Build history of the part. All positions in model axes, mm. A direction names the side the tool comes from. Round coordinates to 2 decimals unless told otherwise and drop trailing zeros. Write each loop counter-clockwise with the first axis right and the second up, starting at its lowest first coordinate (ties: lowest second). Pieces come first, ordered by that corner, then holes.
Item 1: Band-saw the part on C-C, the plane y = -17. Write the cut outline in (x, z), then the cut area to 3 significant figures.
Item 2: Band-saw the part on D-D, the plane y = -1.5. Write the cut outline in (x, z).
Item 3: 3-axis set-ups, long thin cutter, end or side, ignore diameter. For faces 1 (the flat face through (-19.198, 6, -4)), 2 (the flat face through (5, -15.387, 25)), 3 (the flat face through (-16.698, 7, 25)), 4 (the flat face through (7, 9, 0)): which of +Z, -Z, +X, -X, +Y, -Y reach the whole face in a straight line?
Item 4: Mould opens along Y. For faces 5 (the flat face through (7, -12.887, 25)), 6 (the flat face through (-21.698, 4, 22)), 7 (the flat face through (5, -17.887, 25)) say: +Y half, -Y half, draft (parallel to the pull), parting line (faces both ways), or undercut.
Item 5: Drop flat-ended pins along their axis: pin 1 Ø21 at (y, z) = (7.5, 24.5) entering from +X; pin 2 Ø24 at (x, y) = (0, 11.5) entering from +Z; pin 3 Ø1.2 at (y, z) = (13.5, -4) entering from +X. Give the stop position or say it passes through.
Item 6: Band-saw the part on B-B, the plane x = -8. Write the cut outline in (y, z).
Item 7: Band-saw the part on A-A, the plane z = 38. Write the cut outline in (x, y), then the cut area to 4 significant figures.
Item 8: Wall check: probe 1 along Y at (x, z) = (9, 21.5); probe 2 along Z at (x, y) = (8.5, 0.5); probe 3 along X at (y, z) = (6, 41). Give the ranges that are in metal, low to high.
```python
from build123d import *

# Parameters (mm, degrees)
F0_W     = 42.5
F0_H     = 42.5
F0_W_2   = 2.5
F0_H_2   = 2.5
F1_DEPTH = 2.5
F2_DEPTH = 50
F3_W     = 2.5
F3_H     = 47.5
F3_W_2   = 47.5
F3_H_2   = 2.5
F4_DEPTH = 2.5
F5_W     = 47.5
F5_H     = 47.5
F6_DEPTH = 2.5


with BuildPart() as f1:
    # F0 (on Top) → F1 (new body)
    with BuildSketch(Plane.XY):
        with Locations((7.0520306379, 8.3629446477)):
            Rectangle(F0_W, F0_H)
        with Locations((-15.4479693621, 8.3629446477)):
            Rectangle(F0_W_2, F0_H)
        with Locations((-17.9479693621, 8.3629446477)):
            Rectangle(F0_W_2, F0_H)
        with Locations((-20.4479693621, 8.3629446477)):
            Rectangle(F0_W_2, F0_H)
        with Locations((7.0520306379, -14.1370553523)):
            Rectangle(F0_W, F0_H_2)
        with Locations((7.0520306379, -16.6370553523)):
            Rectangle(F0_W, F0_H_2)
        with Locations((7.0520306379, -19.1370553523)):
            Rectangle(F0_W, F0_H_2)
        with Locations((-15.4479693621, -19.1370553523)):
            Rectangle(F0_W_2, F0_H_2)
        with Locations((-17.9479693621, -19.1370553523)):
            Rectangle(F0_W_2, F0_H_2)
        with Locations((-20.4479693621, -19.1370553523)):
            Rectangle(F0_W_2, F0_H_2)
        with Locations((-20.4479693621, -16.6370553523)):
            Rectangle(F0_W_2, F0_H_2)
        with Locations((-17.9479693621, -16.6370553523)):
            Rectangle(F0_W_2, F0_H_2)
        with Locations((-15.4479693621, -16.6370553523)):
            Rectangle(F0_W_2, F0_H_2)
        with Locations((-15.4479693621, -14.1370553523)):
            Rectangle(F0_W_2, F0_H_2)
        with Locations((-17.9479693621, -14.1370553523)):
            Rectangle(F0_W_2, F0_H_2)
        with Locations((-20.4479693621, -14.1370553523)):
            Rectangle(F0_W_2, F0_H_2)
    extrude(amount=-F1_DEPTH)

    # F0 (on Top) → F2 (join)
    with BuildSketch(Plane.XY):
        with Locations((-20.4479693621, 8.3629446477)):
            Rectangle(F0_W_2, F0_H)
        with Locations((-20.4479693621, -14.1370553523)):
            Rectangle(F0_W_2, F0_H_2)
        with Locations((-15.4479693621, 8.3629446477)):
            Rectangle(F0_W_2, F0_H)
        with Locations((-15.4479693621, -14.1370553523)):
            Rectangle(F0_W_2, F0_H_2)
        with Locations((-15.4479693621, -19.1370553523)):
            Rectangle(F0_W_2, F0_H_2)
        with Locations((7.0520306379, -14.1370553523)):
            Rectangle(F0_W, F0_H_2)
        with Locations((-17.9479693621, -19.1370553523)):
            Rectangle(F0_W_2, F0_H_2)
        with Locations((-20.4479693621, -19.1370553523)):
            Rectangle(F0_W_2, F0_H_2)
        with Locations((7.0520306379, -19.1370553523)):
            Rectangle(F0_W, F0_H_2)
        with Locations((-20.4479693621, -16.6370553523)):
            Rectangle(F0_W_2, F0_H_2)
    extrude(amount=F2_DEPTH)

    # F3 (on face) → F4 (join)
    with BuildSketch(Plane(origin=(0, 0, -2.5), x_dir=(1, 0, 0), z_dir=(0, 0, -1))):
        with Locations((-20.4479693621, -5.8629446477)):
            Rectangle(F3_W, F3_H)
        with Locations((4.5520306379, 19.1370553523)):
            Rectangle(F3_W_2, F3_H_2)
        with Locations((-20.4479693621, 19.1370553523)):
            Rectangle(F3_W, F3_H_2)
    extrude(amount=F4_DEPTH)

    # F5 (on face) → F6 (join)
    with BuildSketch(Plane(origin=(0, 0, -5), x_dir=(1, 0, 0), z_dir=(0, 0, -1))):
        with Locations((4.5520306379, -5.8629446477)):
            Rectangle(F5_W, F5_H)
        Polygon((28.3020306379, 20.3870553523), (-21.6979693621, 20.3870553523), (-21.6979693621, -29.6129446477), (-19.1979693621, -29.6129446477), (-19.1979693621, 17.8870553523), (28.3020306379, 17.8870553523), align=None)
    extrude(amount=F6_DEPTH)


solid = f1.part
```
Results:
1. outline: (-21.7, -7.5) - (28.3, -7.5) - (28.3, -5) - (-19.2, -5) - (-19.2, -2.5) - (28.3, -2.5) - (28.3, 0) - (-19.2, 0) - (-19.2, 50) - (-21.7, 50) - close
1. area: 381 mm2
2. outline: (-21.7, -7.5) - (28.3, -7.5) - (28.3, -5) - (-19.2, -5) - (-19.2, -2.5) - (28.3, -2.5) - (28.3, 0) - (-14.2, 0) - (-14.2, 50) - (-16.7, 50) - (-16.7, 0) - (-19.2, 0) - (-19.2, 50) - (-21.7, 50) - close
3. face 1: +X, +Y
3. face 2: +Z, +X
3. face 3: +Z, +Y
3. face 4: +Z, +X, +Y
4. face 5: +Y half
4. face 6: draft
4. face 7: undercut
5. pin 1: stops at x = -14.2
5. pin 2: stops at z = 0
5. pin 3: stops at x = -19.2
6. outline: (-20.39, -7.5) - (29.61, -7.5) - (29.61, -5) - (-17.89, -5) - (-17.89, -2.5) - (29.61, -2.5) - (29.61, 0) - (-12.89, 0) - (-12.89, 50) - (-15.39, 50) - (-15.39, 0) - (-17.89, 0) - (-17.89, 50) - (-20.39, 50) - close
7. outline: (-21.7, -20.39) - (28.3, -20.39) - (28.3, -17.89) - (-19.2, -17.89) - (-19.2, 29.61) - (-21.7, 29.61) - close; (-16.7, -15.39) - (28.3, -15.39) - (28.3, -12.89) - (-14.2, -12.89) - (-14.2, 29.61) - (-16.7, 29.61) - close
7. area: 462.5 mm2
8. probe 1: y = -20.39 to -17.89, -15.39 to -12.89
8. probe 2: z = -7.5 to -5, -2.5 to 0
8. probe 3: x = -21.7 to -19.2, -16.7 to -14.2
